Autodesk Inventor part; units mm, degrees
ref_plane "YZ Plane" through (0, 0, 0) normal (1, 0, 0) x (0, 1, 0)
ref_plane "XZ Plane" through (0, 0, 0) normal (0, 1, 0) x (-1, 0, 0)
ref_plane "XY Plane" through (0, 0, 0) normal (0, 0, 1) x (1, 0, 0)
sketch "Boceto1" plane through (0, 0, 0) normal (0, 1, 0) x (-1, 0, 0)
  line L0 (-382.6667, -300) -> (-382.6667, -100)
  line L1 (-382.6667, -300) -> (-382.6667, -233.3333)
  line L2 (-382.6667, -233.3333) -> (-382.6667, -300)
  line L3 (-382.6667, -300) -> (-364.7679, -401.509)
  line L4 (-382.6667, -300) -> (-382.6667, -100)
  line L5 (-382.6667, -100) -> (-364.7679, 1.509)
  line L6 (-376, -300) -> (-376, -100)
  line L7 (-376.1013, -298.8423) -> (-357.9984, -401.509)
  line L8 (-376.1013, -101.1577) -> (-357.9984, 1.509)
  line L9 (-357.9984, 1.509) -> (-364.7679, 1.509)
  line L10 (-357.9984, -401.509) -> (-364.7679, -401.509)
  point P0 (0, 0)
  point P1 (-376, -299.4167)
  point P2 (-376, -100.5833)
  dimension "d14" = 200
extrude "Extrusión1" add sketch "Boceto1" along normal blind 80
properties part number "guia"
Geometry check sheet. Reference: the model listing, model coordinates, mm. A direction names the side the tool comes from. Round coordinates to 2 decimals unless told otherwise and drop trailing zeros. Write each loop counter-clockwise with the first axis right and the second up, starting at its lowest first coordinate (ties: lowest second). Pieces come first, ordered by that corner, then holes. Notation, with made-up numbers: (-13.75, 46.5) -> (9.25, 46.5) arc R21 cw to (9.25, 83.5) -> close; hole circle Ø5 at (-19, 43.5). An arc over 180 degrees is marked (long way). One line per item, written item: value. Start each with the question number.
(1) Access from +Z, -Z, +X, -X, +Y, -Y to the whole of each face (thin tool, end or side, straight path). Record for faces 1 (the flat face through (361, 39, -401.509)), 2 (the flat face through (367.125, 39.44, -349.748)).
(2) Cross-section at B-B, the plane z = -242. Record the cut outline in (x, y), and give its area (3 significant figures).
(3) Cross-section at C-C, the plane z = -359. Record the cut outline in (x, y), and give its area (3 significant figures).
(4) Cross-section at A-A, the plane y = 39. Record the cut outline in (x, z).
(5) Go/stop test with flat-tipped pins: pin 1 Ø4 at (y, z) = (46.5, -216.5) entering from -X; pin 2 Ø2 at (y, z) = (35, -59) entering from -X; pin 3 Ø1.5 at (y, z) = (13.5, -340.5) entering from +X. Record where each tip stops, or that it passes through.
(6) Draft check along Z on faces 3 (the flat face through (382, 0, -199)), 4 (the flat face through (361, 39, 1.509)), 5 (the flat face through (376, 39, -201)). Enter one of: +Z half, -Z half, draft (parallel to the pull), parting line (faces both ways), or undercut.
(7) Scan lines: line 1 (X direction, y = 68, z = -267); line 2 (X direction, y = 16.5, z = -369). Record each from-to range of solid material in increasing order. Write a range as [from, to].
Answer:
1. face 1: -Z, +X, -X, +Y, -Y
1. face 2: -X, +Y, -Y
2. outline: (376, 0) -> (382.67, 0) -> (382.67, 80) -> (376, 80) -> close
2. area: 533 mm²
3. outline: (365.49, 0) -> (372.26, 0) -> (372.26, 80) -> (365.49, 80) -> close
3. area: 542 mm²
4. outline: (358, -401.51) -> (364.77, -401.51) -> (382.67, -300) -> (382.67, -100) -> (364.77, 1.51) -> (358, 1.51) -> (376, -100.58) -> (376, -299.42) -> close
5. pin 1: x = 376
5. pin 2: x = 368.49
5. pin 3: x = 375.66
6. face 3: draft
6. face 4: +Z half
6. face 5: undercut
7. line 1: [376, 382.67]
7. line 2: [363.73, 370.5]
